```python
from build123d import *

# Parameters (mm, degrees)
SKETCH1_R           = 76.2
SKETCH1_R_2         = 74.7776
BOSS_EXTRUDE1_DEPTH = 101.6
SKETCH2_R           = 6.35
CUT_EXTRUDE1_DEPTH  = 5.08
CIRPATTERN1_COUNT   = 4


with BuildPart() as part:
    # Sketch1 → Boss-Extrude1 (new, symmetric)
    with BuildSketch(Plane(origin=(0, 0, 0), x_dir=(1, 0, 0), z_dir=(0, 1, 0))):
        with Locations(Location((0, 0, 0), (0, 0, 270))):
            Circle(SKETCH1_R)
        with Locations(Location((0, 0, 0), (0, 0, 270))):
            Circle(SKETCH1_R_2, mode=Mode.SUBTRACT)
    extrude(amount=BOSS_EXTRUDE1_DEPTH, both=True)

    # Sketch2 → Cut-Extrude1 (cut)
    with BuildSketch(Plane(origin=(54.887325412, 0, -54.887325412), x_dir=(0, -1, 0), z_dir=(0.7071067811865488, 0, -0.7071067811865464))):
        with Locations(Location((0, 0, 0), (0, 0, 90))):
            Circle(SKETCH2_R)
    cut_extrude1 = extrude(amount=-CUT_EXTRUDE1_DEPTH, mode=Mode.SUBTRACT)

    # CirPattern1: Cut-Extrude1 ×4 about axis
    cirpattern1_axis = Axis((0, 0, 0), (0, 1, 0))
    for i in range(1, CIRPATTERN1_COUNT):
        add(cut_extrude1.rotate(cirpattern1_axis, i * 360 / CIRPATTERN1_COUNT), mode=Mode.SUBTRACT)


solid = part.part
```
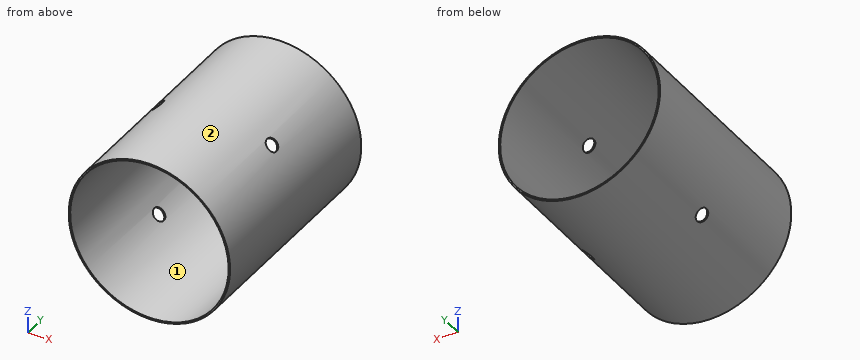
The listing builds one solid part. Answer for the finished solid, in the listing's coordinates (mm). Face numbers are marked on the shaded views. Round coordinates to 2 decimals unless told otherwise and drop trailing zeros. Loops run counter-clockwise (first coordinate to the right, second up) from the corner with the lowest first, then second, coordinate; pieces in that order, holes last.
Q1. For a pull along X with two mould halves and no side action, classify the marked faces 1 and 2 as released by +X, released by -X, zero draft, split by the parting line, or undercut.
Q2. Section A-A, the plane x = 0 is taken. Determine the outline of the cut face in (y, z).
Q3. Section C-C, the plane y = 69.5 is taken. Determine the outline of the cut face in (x, z), then the cut area to 3 significant figures.
Q4. Section B-B, the plane z = 62 is taken. Determine the outline of the cut face in (x, y), then the cut area to 3 significant figures.
Q5. Find the intervals of material crossed by line 1 (Z direction, x = -2, y = -31.5); line 2 (X direction, y = -42.5, z = 0); line 3 (X direction, y = -22, z = -59), in increasing order.
Q6. Given pin 1 Ø5 at (y, z) = (-34.5, -31) entering from -X; pin 2 Ø1.5 at (x, y) = (13.5, -70.5) entering from +Z; pin 3 Ø5 at (y, z) = (49.5, -17) entering from -X, each flat-ended and moving along its own axis, determine where each tip first touches the part or whether it passes through.
Completed:
1. face 1: undercut
1. face 2: split by the parting line
2. outline: (-101.6, -76.2) - (101.6, -76.2) - (101.6, -74.78) - (-101.6, -74.78) - close; (-101.6, 74.78) - (101.6, 74.78) - (101.6, 76.2) - (-101.6, 76.2) - close
3. outline: circle Ø152.4 at (0, 0); hole circle Ø149.56 at (0, 0)
3. area: 675 mm2
4. outline: (-44.3, -101.6) - (-41.81, -101.6) - (-41.81, 101.6) - (-44.3, 101.6) - close; (41.81, -101.6) - (44.3, -101.6) - (44.3, 101.6) - (41.81, 101.6) - close
4. area: 1,010 mm2
5. line 1: z = -76.17 to -74.75, 74.75 to 76.17
5. line 2: x = -76.2 to -74.78, 74.78 to 76.2
5. line 3: x = -48.22 to -45.94, 45.94 to 48.22
6. pin 1: stops at x = -70.67
6. pin 2: stops at z = 75.13
6. pin 3: stops at x = -74.81
